The listing builds one solid part. Answer for the finished solid, in the listing's coordinates (mm). A direction names the side the tool comes from. Round coordinates to 2 decimals unless told otherwise and drop trailing zeros. Order: outer loops, then holes, each group sorted by start corner. A loop starts at its lowest first (then second) coordinate and runs counter-clockwise, first axis right, second up. Notation, with made-up numbers: (15, 56) -> (48, 56) arc R18 ccw to (48, 80) -> close; hole circle Ø6 at (-13.75, 20.5). An arc over 180 degrees is marked (long way). Return JSON: item names as keys, results as strings. Group by question number.
(1) Consider line 1 (Y direction, x = 80, z = 2.45); line 2 (X direction, y = -22, z = 1.75); line 3 (Y direction, x = 71, z = 0.75). Determine where each line is inside the solid, lowest interval first. Write a range as [from, to].
(2) The part is cut by section A-A (y = -19.05). Determine the outline of the cut face in (x, z), plus the area to 3 significant figures.
(3) Each of these flat-tipped pins is pushed along its axis until it touches: pin 1 (1.5 mm diameter, centred on y = -7.5, z = 2, fed in from +X); pin 2 (0.9 mm diameter, centred on x = 58.5, z = 2, fed in from -Y); pin 3 (0.9 mm diameter, centred on y = -33, z = 1, fed in from -X). Where does it stop, or does it pass through?
(4) Which of the six approach directions +Z, -Z, +X, -X, +Y, -Y give full straight-line access (tool end or side, diameter ignored) to faces 5 (the face through (79, -26.67, 1)), 6 (the face through (109, -31.75, 1)), 7 (the face through (62, -31.75, 1)), 8 (the face through (74.435, -29, 1)), 9 (the face through (113, -6.35, 1))?
(5) Determine the mould class of faces 1 (the face through (84, -31.75, 1)), 2 (the face through (72.072, -24, 1)), 3 (the face through (76, -21.59, 1)), 4 (the face through (114.3, -19, 1)) for opening direction Y: +Y half, -Y half, draft (parallel to the pull), parting line (faces both ways), or undercut.
(6) The part is cut by section C-C (x = 88.5). Determine the outline of the cut face in (y, z).
from build123d import *

# Parameters (mm, degrees)
SKETCH1_R           = 1.7526
BOSS_EXTRUDE1_DEPTH = 3


with BuildPart() as part:
    # Sketch1 → Boss-Extrude1 (new body)
    with BuildSketch(Plane.XY):
        Polygon((49.628328589, 31.75), (111.125, 31.75), (114.475, 31.75), (114.475, 19.05), (111.3, 19.05), (111.3, -6.35), (114.3, -6.35), (114.3, -18.229405084), (114.3, -19.870594916), (114.3, -31.75), (111.125, -31.75), (102.87, -31.75), (102.87, -34.75), (90.17, -34.75), (90.17, -31.75), (88.19515, -31.75), (77.9653, -31.75), (77.9653, -26.67), (80.3275, -26.67), (80.3275, -21.59), (72.0725, -21.59), (72.0725, -26.67), (74.4347, -26.67), (74.4347, -31.75), (49.628328589, -31.75), align=None)
        with Locations((112.395, -19.05)):
            Circle(SKETCH1_R, mode=Mode.SUBTRACT)
    extrude(amount=BOSS_EXTRUDE1_DEPTH)


solid = part.part
Answer below:
{
 "1": {"line 1": "y = [-31.75, -26.67], [-21.59, 31.75]", "line 2": "x = [49.63, 72.07], [80.33, 114.3]", "line 3": "y = [-31.75, 31.75]"},
 "2": {"outline": "(49.63, 0) -> (110.64, 0) -> (110.64, 3) -> (49.63, 3) -> close; (114.15, 0) -> (114.3, 0) -> (114.3, 3) -> (114.15, 3) -> close", "area": "183 mm²"},
 "3": {"pin 1": "stops at x = 114.3", "pin 2": "stops at y = -31.75", "pin 3": "stops at x = 90.17"},
 "4": {"face 5": "+Z, -Z", "face 6": "+Z, -Z, +X, -Y", "face 7": "+Z, -Z, -X, -Y", "face 8": "+Z, -Z, -Y", "face 9": "+Z, -Z, +X"},
 "5": {"face 1": "-Y half", "face 2": "undercut", "face 3": "undercut", "face 4": "draft"},
 "6": {"outline": "(-31.75, 0) -> (31.75, 0) -> (31.75, 3) -> (-31.75, 3) -> close"}
}
